```python
from build123d import *

# Parameters (mm, degrees)
BOSS_EXTRUDE1_DEPTH  = 4.5
SKETCH2_W            = 9
SKETCH2_H            = 10
BOSS_EXTRUDE2_DEPTH  = 4.5
BOSS_EXTRUDE3_DEPTH  = 4.5
CUT_EXTRUDE1_DEPTH   = 84.792899461
SKETCH5_W            = 10
SKETCH5_H            = 4.5
BOSS_EXTRUDE4_DEPTH  = 4.5
CUT_EXTRUDE4_DEPTH   = 84.792899461
BOSS_EXTRUDE11_DEPTH = 4.5
SKETCH21_R           = 1.55
CUT_EXTRUDE8_DEPTH   = 86.089658596
SKETCH22_R           = 13.25
CUT_EXTRUDE9_DEPTH   = 86.089658596


with BuildPart() as part:
    # Sketch1 → Boss-Extrude1 (new body)
    with BuildSketch(Plane(origin=(0, 0, 0), x_dir=(0, 0, -1), z_dir=(1, 0, 0))):
        Polygon((0, 0), (0, -35), (-76, 0), align=None)
    extrude(amount=BOSS_EXTRUDE1_DEPTH)

    # Sketch2 → Boss-Extrude2 (add, through all)
    with BuildSketch(Plane(origin=(4.5, 0, 0), x_dir=(0, 0, -1), z_dir=(1, 0, 0))):
        with Locations((0, -7.5)):
            Rectangle(SKETCH2_W, SKETCH2_H)
    extrude(amount=-BOSS_EXTRUDE2_DEPTH)

    # Sketch3 → Boss-Extrude3 (add, through all)
    with BuildSketch(Plane(origin=(4.5, 0, 0), x_dir=(0, 0, -1), z_dir=(1, 0, 0))):
        Polygon((0, -35), (-40, -35), (-76, 0), (0, -25), align=None)
    extrude(amount=-BOSS_EXTRUDE3_DEPTH)

    # Sketch4 → Cut-Extrude1 (cut, through all)
    with BuildSketch(Plane(origin=(4.5, 0, 0), x_dir=(0, 0, -1), z_dir=(1, 0, 0))):
        with BuildLine():
            Line((0, -31.25), (0, -27.75))
            Line((0, -27.75), (-3.8, -27.75))
            Line((-3.8, -27.75), (-3.8, -26.75))
            ThreePointArc((-3.8, -26.75), (-3.873223305, -26.573223305), (-4.05, -26.5))
            Line((-4.05, -26.5), (-7.75, -26.5))
            ThreePointArc((-7.75, -26.5), (-7.926776695, -26.573223305), (-8, -26.75))
            Line((-8, -26.75), (-8, -27.75))
            Line((-8, -27.75), (-10.5, -27.75))
            Line((-10.5, -27.75), (-10.5, -31.25))
            Line((-10.5, -31.25), (-8, -31.25))
            Line((-8, -31.25), (-8, -32.25))
            ThreePointArc((-8, -32.25), (-7.926776695, -32.426776695), (-7.75, -32.5))
            Line((-7.75, -32.5), (-4.05, -32.5))
            ThreePointArc((-4.05, -32.5), (-3.873223305, -32.426776695), (-3.8, -32.25))
            Line((-3.8, -32.25), (-3.8, -31.25))
            Line((-3.8, -31.25), (0, -31.25))
        make_face()
    extrude(amount=-CUT_EXTRUDE1_DEPTH, mode=Mode.SUBTRACT)

    # Sketch5 → Boss-Extrude4 (add, through all)
    with BuildSketch(Plane(origin=(4.5, 0, 0), x_dir=(0, 0, -1), z_dir=(1, 0, 0))):
        with Locations((-20, 2.25)):
            Rectangle(SKETCH5_W, SKETCH5_H)
        with Locations((-40, 2.25)):
            Rectangle(SKETCH5_W, SKETCH5_H)
    extrude(amount=-BOSS_EXTRUDE4_DEPTH)

    # Sketch11 → Cut-Extrude4 (cut, through all)
    with BuildSketch(Plane.ZY):
        with BuildLine():
            Line((5.75, -10.5), (9.25, -10.5))
            Line((9.25, -10.5), (9.25, -8))
            Line((9.25, -8), (10.25, -8))
            ThreePointArc((10.25, -8), (10.426776695, -7.926776695), (10.5, -7.75))
            Line((10.5, -7.75), (10.5, -4.05))
            ThreePointArc((10.5, -4.05), (10.426776695, -3.873223305), (10.25, -3.8))
            Line((10.25, -3.8), (9.25, -3.8))
            Line((9.25, -3.8), (9.25, 0))
            Line((9.25, 0), (5.75, 0))
            Line((5.75, 0), (5.75, -3.8))
            Line((5.75, -3.8), (4.75, -3.8))
            ThreePointArc((4.75, -3.8), (4.573223305, -3.873223305), (4.5, -4.05))
            Line((4.5, -4.05), (4.5, -7.75))
            ThreePointArc((4.5, -7.75), (4.573223305, -7.926776695), (4.75, -8))
            Line((4.75, -8), (5.75, -8))
            Line((5.75, -8), (5.75, -10.5))
        make_face()
    extrude(amount=-CUT_EXTRUDE4_DEPTH, mode=Mode.SUBTRACT)

    # Sketch20 → Boss-Extrude11 (add, through all)
    with BuildSketch(Plane(origin=(4.5, 0, 0), x_dir=(0, 0, -1), z_dir=(1, 0, 0))):
        with BuildLine():
            Line((-9, -38), (-58.008074506, -38))
            ThreePointArc((-58.008074506, -38), (-59.667515225, -37.499251188), (-60.772980632, -36.164171))
            Line((-60.772980632, -36.164171), (-76, 0))
            Line((-76, 0), (-40, -35))
            Line((-40, -35), (-6, -35))
            Line((-6, -35), (-9, -38))
        make_face()
    extrude(amount=-BOSS_EXTRUDE11_DEPTH)

    # Sketch21 → Cut-Extrude8 (cut, through all)
    with BuildSketch(Plane(origin=(4.5, 0, 0), x_dir=(0, 0, -1), z_dir=(1, 0, 0))):
        with Locations((-51, -34.5)):
            Circle(SKETCH21_R)
        with Locations((-26, -34.5)):
            Circle(SKETCH21_R)
    extrude(amount=-CUT_EXTRUDE8_DEPTH, mode=Mode.SUBTRACT)

    # Sketch22 → Cut-Extrude9 (cut, through all)
    with BuildSketch(Plane(origin=(4.5, 0, 0), x_dir=(0, 0, -1), z_dir=(1, 0, 0))):
        with Locations((-52, -18)):
            Circle(SKETCH22_R)
    extrude(amount=-CUT_EXTRUDE9_DEPTH, mode=Mode.SUBTRACT)


solid = part.part
```
Read the model definition and answer for the solid it produces. Units are mm, in the model's axes. A direction names the side the tool comes from. Coordinates: 2 decimals unless noted, no trailing zeros. Write each loop counter-clockwise with the first axis right and the second up, starting at its lowest first coordinate (ties: lowest second). Pieces come first, ordered by that corner, then holes. Notation, with made-up numbers: (2, 7.25) -> (9, 7.25) arc R25 ccw to (9, 45.25) -> close; hole circle Ø4 at (48.5, 3). An arc over 180 degrees is marked (long way). Return JSON: item names as keys, results as strings.
1. A cutting plane is placed at D-D (z = 51). Determine the outline of the cut face in (x, y).
Found:
{"outline": "(0, -38) -> (4.5, -38) -> (4.5, -36.05) -> (0, -36.05) -> close; (0, -32.95) -> (4.5, -32.95) -> (4.5, -31.21) -> (0, -31.21) -> close; (0, -4.79) -> (4.5, -4.79) -> (4.5, 0) -> (0, 0) -> close"}
2. Each of these flat-tipped pins is pushed along its axis until it touches: P1, Ø1.5, axis at x = 3, y = -21, coming from the +Z side; P2, Ø1.8, axis at x = 2, y = -29, coming from the -Z side; P3, Ø1, axis at x = 3, y = -19.5, coming from the +Z side. Where does it stop, or does it pass through?
Found:
{"P1": "z = 67.47", "P2": "z = 10.5", "P3": "z = 68"}
3. Find the intervals of material crossed by line 1 along Y through (x, z) = (1.4, 26); line 2 along Y through (x, z) = (2.05, 52); line 3 along Z through (x, y) = (1.4, -9.5), in increasing order. Write a range as from..to.
Found:
{"line 1": "-38..-36.05, -32.95..0", "line 2": "-38..-35.68, -33.32..-31.25, -4.75..0", "line 3": "-4.5..5.75, 9.25..41.84, 62.16..72"}
4. A cutting plane is placed at B-B (y = -30). Determine the outline of the cut face in (x, z).
Found:
{"outline": "(0, 10.5) -> (4.5, 10.5) -> (4.5, 46.38) -> (0, 46.38) -> close; (0, 57.62) -> (4.5, 57.62) -> (4.5, 63.37) -> (0, 63.37) -> close"}
5. A cutting plane is placed at C-C (x = 1.1). Give the number of separate pieces and of enclosed holes in the cut face, and give its area (3 significant figures).
Found:
{"separate pieces": "1", "enclosed holes": "3", "area": "2,030 mm2"}
6. Determine the mould class of faces 1 (the face through (2, -35, 3)), 2 (the face through (2, -33, 0)), 3 (the face through (2, -26.5, 6)), 4 (the face through (2.282, -34.034, 49.522)) for opening direction Y: pulls with the +Y half, pulls with the -Y half, needs draft (parallel to the pull), parting line crosses it, or undercut.
Found:
{"face 1": "pulls with the -Y half", "face 2": "needs draft", "face 3": "undercut", "face 4": "undercut"}
7. A cutting plane is placed at A-A (z = 26). Determine the outline of the cut face in (x, y).
Found:
{"outline": "(0, -38) -> (4.5, -38) -> (4.5, -36.05) -> (0, -36.05) -> close; (0, -32.95) -> (4.5, -32.95) -> (4.5, 0) -> (0, 0) -> close"}
8. A tool of negligible diameter and unlimited length cuts with its end or side. For faces 5 (the face through (2, 2, 45)), 6 (the face through (2, -9, 9.25)), 7 (the face through (2, -27.75, 2)), 8 (the face through (2, 0, 12)), 9 (the face through (2, -38, 33)), from which of +Z, -Z, +X, -X, +Y, -Y can it reach the whole face along a straight path? Write none if from no direction.
Found:
{"face 5": "+Z, +X, -X, +Y", "face 6": "+X, -X, +Y", "face 7": "-Z, +X, -X", "face 8": "-Z, +X, -X, +Y", "face 9": "+Z, -Z, +X, -X, -Y"}
